The model under review builds one solid part; all positions refer to its coordinate system, in mm. Round coordinates to 2 decimals unless told otherwise and drop trailing zeros. Order: outer loops, then holes, each group sorted by start corner. A loop starts at its lowest first (then second) coordinate and runs counter-clockwise, first axis right, second up. Notation, with made-up numbers: M 73.5,81.5 L 79.5,81.5 A25 ccw 79.5,93.5 Z; hole C 30,50 d10. An arc over 180 degrees is marked long. Answer as a JSON object with one key per item and string values. Group by question number.
1) Consider section C-C, the plane z = 27. Write out the cut boundary in (x, y).
2) The part is to be moulded in two halves that separate along X. For faces 1 (the cylindrical face through (-23.951, -0.178, -49.272)), 2 (the cylindrical face through (-19.787, -0.178, -38.07)), 3 (the flat face through (0, 0, -50.8)), say which applies: +X half, -X half, draft (parallel to the pull), parting line (faces both ways), or undercut.
3) Consider section B-B, the plane z = 38. Write out the cut boundary in (x, y).
4) To check wall thickness, follow line 1 (X direction, y = 3.75, z = 41); line 2 (Z direction, x = -3, y = 0.25); line 3 (X direction, y = 6.5, z = 43.5). State the ranges of each line that lie inside material, in increasing order.
5) Consider section A-A, the plane x = 0. Write out the cut boundary in (y, z), then the cut area to 3 significant figures.
6) Consider section D-D, the plane y = -5.5. Write out the cut boundary in (x, z), then the cut area to 3 significant figures.
7) Insertion check: pin 1 Ø14 at (x, z) = (-16.54, -41.05) entering from -Y. The pin has a flat end and moves straight along its axis. Give the tip position at first contact, or say it passes through.
```python
from build123d import *

# Parameters (mm, degrees)
F0_W     = 50.8
F0_H     = 101.6
F0_R     = 7.62
F1_DEPTH = 12.7
F2_R     = 5.08
F3_R     = 4.408168
F4_DEPTH = 25.401


with BuildPart() as f1:
    # F0 (on Front) → F1 (new body, symmetric)
    with BuildSketch(Plane.XZ):
        Rectangle(F0_W, F0_H)
        with Locations((0, -22.179579)):
            Circle(F0_R, mode=Mode.SUBTRACT)
        with Locations((0, 22.179579)):
            Circle(F0_R, mode=Mode.SUBTRACT)
    extrude(amount=F1_DEPTH, both=True)

    # F2
    f2_edges = [f1.edges().sort_by_distance(p)[0] for p in [
        (-25.4, 0, 50.8),
        (25.4, 0, 50.8),
        (25.4, 0, -50.8),
        (-25.4, 0, -50.8),
    ]]
    fillet(f2_edges, radius=F2_R)

    # F3 (on face) → F4 (cut, through all)
    with BuildSketch(Plane.XZ.offset(12.7)):
        with Locations((-16.53761, 41.049208)):
            Circle(F3_R)
        with Locations((16.53761, 41.049208)):
            Circle(F3_R)
        with Locations((16.53761, -41.049208)):
            Circle(F3_R)
        with Locations((-16.53761, -41.049208)):
            Circle(F3_R)
    extrude(amount=-F4_DEPTH, mode=Mode.SUBTRACT)


solid = f1.part
```
Results list:
{
 "1": {"outline": "M -25.4,-12.7 L -5.9,-12.7 L -5.9,12.7 L -25.4,12.7 Z; M 5.9,-12.7 L 25.4,-12.7 L 25.4,12.7 L 5.9,12.7 Z"},
 "2": {"face 1": "-X half", "face 2": "undercut", "face 3": "draft"},
 "3": {"outline": "M -25.4,-12.7 L -19.72,-12.7 L -19.72,12.7 L -25.4,12.7 Z; M -13.35,-12.7 L 13.35,-12.7 L 13.35,12.7 L -13.35,12.7 Z; M 19.72,-12.7 L 25.4,-12.7 L 25.4,12.7 L 19.72,12.7 Z"},
 "4": {"line 1": "-25.4 to -20.95, -12.13 to 12.13, 20.95 to 25.4", "line 2": "-50.8 to -29.18, -15.17 to 15.17, 29.18 to 50.8", "line 3": "-25.4 to -20.2, -12.87 to 12.87, 20.2 to 25.4"},
 "5": {"outline": "M -12.7,-50.8 L 12.7,-50.8 L 12.7,-29.8 L -12.7,-29.8 Z; M -12.7,-14.56 L 12.7,-14.56 L 12.7,14.56 L -12.7,14.56 Z; M -12.7,29.8 L 12.7,29.8 L 12.7,50.8 L -12.7,50.8 Z", "area": "1,810 mm^2"},
 "6": {"outline": "M -25.4,-45.72 A5.08 ccw -20.32,-50.8 L 20.32,-50.8 A5.08 ccw 25.4,-45.72 L 25.4,45.72 A5.08 ccw 20.32,50.8 L -20.32,50.8 A5.08 ccw -25.4,45.72 Z; hole C -16.54,-41.05 d8.82; hole C -16.54,41.05 d8.82; hole C 0,-22.18 d15.24; hole C 0,22.18 d15.24; hole C 16.54,-41.05 d8.82; hole C 16.54,41.05 d8.82", "area": "4,530 mm^2"},
 "7": {"pin 1": "y = -12.7"}
}
